Geometry: see drawing. Coordinates: mm, zero at the bounding-box minimum. A direction names the side the tool comes from. Round coordinates to 2 decimals unless told otherwise and drop trailing zeros. Write each loop counter-clockwise with the first axis right and the second up, starting at its lowest first coordinate (ties: lowest second). Pieces come first, ordered by that corner, then holes.
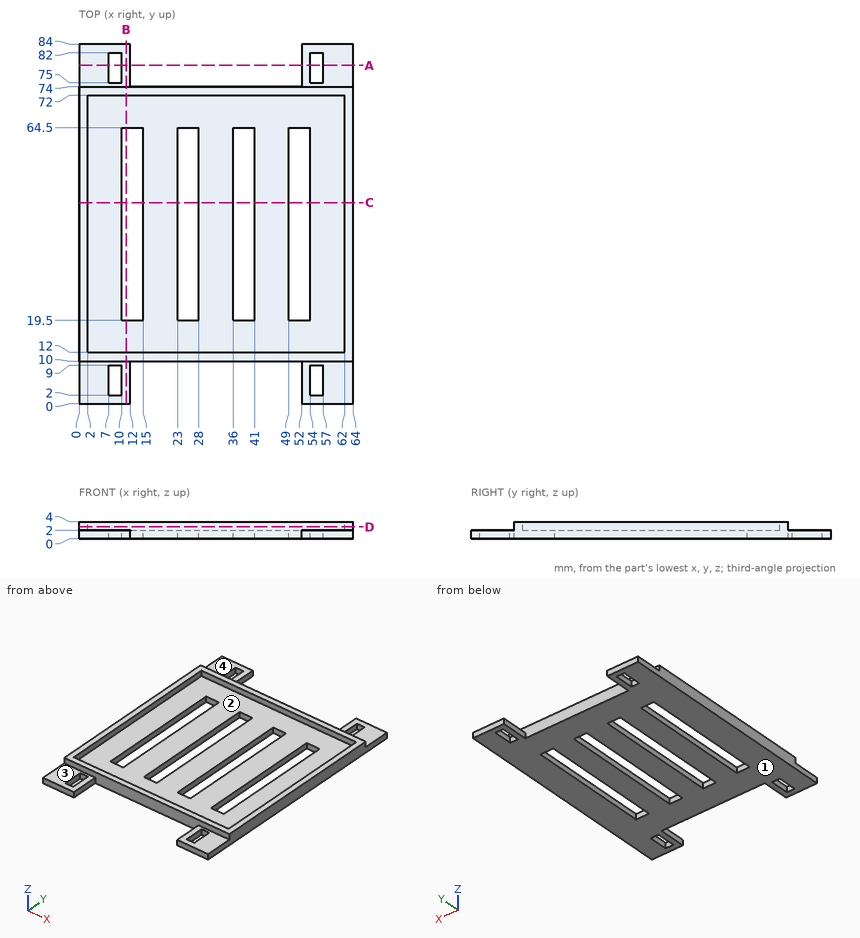
1) Section query A-A on y = 79. Return the cut outline in (x, z).
Taken from the geometry:
outline: (0, 0) - (7, 0) - (7, 2) - (0, 2) - close; (10, 0) - (12, 0) - (12, 2) - (10, 2) - close; (52, 0) - (54, 0) - (54, 2) - (52, 2) - close; (57, 0) - (64, 0) - (64, 2) - (57, 2) - close
2) Material intervals for line 1 (Y direction, x = 8, z = 3.2); line 2 (X direction, y = 54, z = 2.65); line 3 (Y direction, x = 38, z = 1.1), sorted ascending.
Taken from the geometry:
line 1: y = 10 to 12, 72 to 74
line 2: x = 0 to 2, 62 to 64
line 3: y = 10 to 19.5, 64.5 to 74
3) Reachability of the marked faces 3 and 4 from +Z, -Z, +X, -X, +Y, -Y: full face, straight path, thin tool, end or side. Return the list, or none.
Taken from the geometry:
face 3: +Z, +X, -X, -Y
face 4: +Z, +X, -X, +Y
4) Pull-direction query (X, two-part tool) for the marked faces 1 and 2; classes: released by +X, released by -X, zero draft, split by the parting line, or undercut.
Taken from the geometry:
face 1: zero draft
face 2: undercut
5) Contact query for flat-ended pins moving along their axis: P1, Ø1, axis at x = 29.5, z = 3.5, coming from the -Y side; P2, Ø11, axis at x = 6.5, y = 79, coming from the +Z side; P3, Ø1, axis at x = 37, z = 2, coming from the +Y side. Output: stop coordinate, or through.
Taken from the geometry:
P1: stops at y = 10
P2: stops at z = 4
P3: stops at y = 74
6) Section query D-D on z = 2.85. Return the cut outline in (x, y), then the cut area to 3 significant figures.
Taken from the geometry:
outline: (0, 10) - (64, 10) - (64, 74) - (0, 74) - close; hole (2, 12) - (62, 12) - (62, 72) - (2, 72) - close
area: 496 mm2
7) Section query C-C on y = 47. Return the cut outline in (x, z).
Taken from the geometry:
outline: (0, 0) - (10, 0) - (10, 2) - (2, 2) - (2, 4) - (0, 4) - close; (15, 0) - (23, 0) - (23, 2) - (15, 2) - close; (28, 0) - (36, 0) - (36, 2) - (28, 2) - close; (41, 0) - (49, 0) - (49, 2) - (41, 2) - close; (54, 0) - (64, 0) - (64, 4) - (62, 4) - (62, 2) - (54, 2) - close
8) Section query B-B on x = 11. Return the cut outline in (y, z), then the cut area to 3 significant figures.
Taken from the geometry:
outline: (0, 0) - (19.5, 0) - (19.5, 2) - (12, 2) - (12, 4) - (10, 4) - (10, 2) - (0, 2) - close; (64.5, 0) - (84, 0) - (84, 2) - (74, 2) - (74, 4) - (72, 4) - (72, 2) - (64.5, 2) - close
area: 86.0 mm2
